Design review of the part shown in the three views and the two pictorial views. Dimensions are in mm from the part's minimum x, y and z. Give positions to 0.01 mm unless a question says otherwise; leave off trailing zeros. Order: outer loops, then holes, each group sorted by start corner. A loop starts at its lowest first (then second) coordinate and runs counter-clockwise, first axis right, second up.
Item 1: For probe 1 along X at (y, z) = (22.75, 1.15); probe 2 along Y at (x, z) = (14.5, 0.2); probe 3 along X at (y, z) = (29, 1.2), list the stretches that pass through material, from the lowest coordinate up.
Item 2: Consider section A-A (y = 16.25). Give the boundary of the cut face in (x, z).
Item 3: Consider section C-C (x = 2). Give the boundary of the cut face in (y, z), plus the area to 3 significant figures.
Item 4: For P1, Ø1.6, axis at x = 15, z = 1, coming from the +Y side, flat-tipped, find the tip position at first contact; note if it passes through.
Item 5: Consider section D-D (y = 27.75). Give the boundary of the cut face in (x, z), plus the area to 3 significant figures.
Item 6: Consider section B-B (z = 0.4). Give the boundary of the cut face in (x, y), plus the area to 3 significant figures.
Item 7: The part is to be moulded in two halves that separate along X. For the marked faces 1, 2, 3 and 4, say which applies: released by +X, released by -X, zero draft, split by the parting line, or undercut.
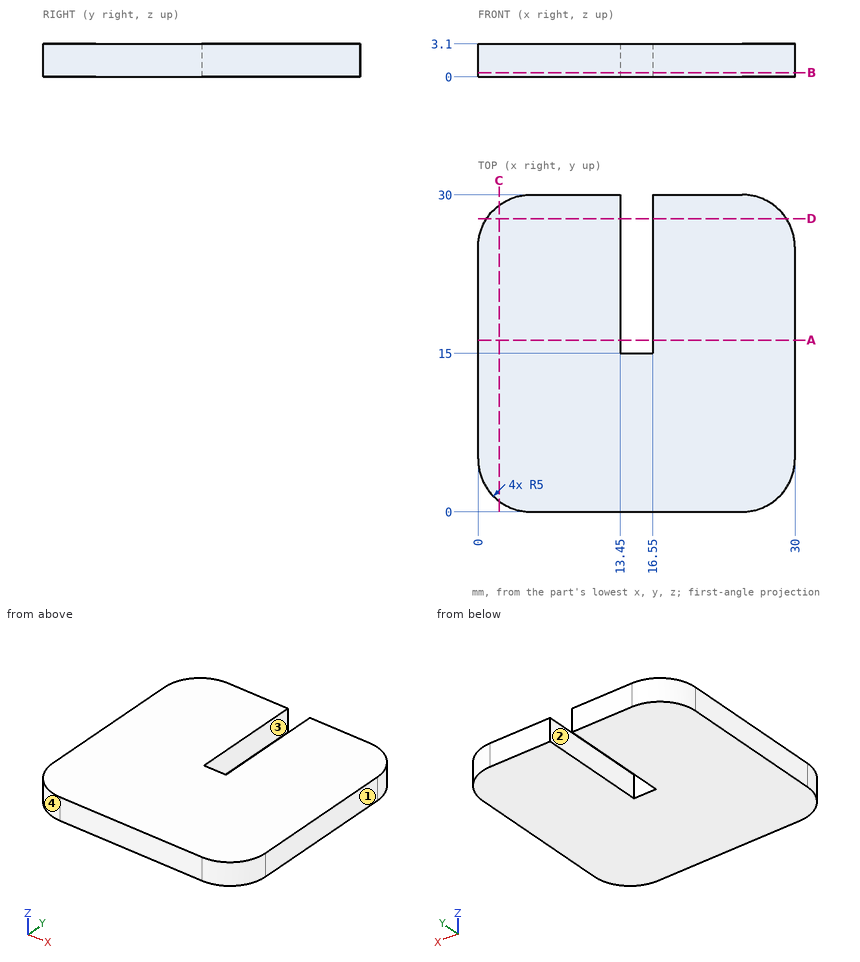
Resolved:
1. probe 1: x = 0 to 13.45, 16.55 to 30
1. probe 2: y = 0 to 15
1. probe 3: x = 2 to 13.45, 16.55 to 28
2. outline: (0, 0) - (13.45, 0) - (13.45, 3.1) - (0, 3.1) - close; (16.55, 0) - (30, 0) - (30, 3.1) - (16.55, 3.1) - close
3. outline: (1, 0) - (29, 0) - (29, 3.1) - (1, 3.1) - close
3. area: 86.8 mm2
4. P1: stops at y = 15
5. outline: (0.82, 0) - (13.45, 0) - (13.45, 3.1) - (0.82, 3.1) - close; (16.55, 0) - (29.18, 0) - (29.18, 3.1) - (16.55, 3.1) - close
5. area: 78.3 mm2
6. outline: (0, 5) arc R5 ccw to (5, 0) - (25, 0) arc R5 ccw to (30, 5) - (30, 25) arc R5 ccw to (25, 30) - (16.55, 30) - (16.55, 15) - (13.45, 15) - (13.45, 30) - (5, 30) arc R5 ccw to (0, 25) - close
6. area: 832 mm2
7. face 1: released by +X
7. face 2: undercut
7. face 3: undercut
7. face 4: released by -X
